Source: CAD feature listing. Evaluate the final solid. Frame: model axes, mm. Face numbers are marked on the shaded views. A direction names the side the tool comes from. Round coordinates to 2 decimals unless told otherwise and drop trailing zeros. Order: outer loops, then holes, each group sorted by start corner. A loop starts at its lowest first (then second) coordinate and runs counter-clockwise, first axis right, second up. Notation, with made-up numbers: (54, 23) - (113, 23) arc R13 ccw to (113, 37) - close; hole circle Ø5 at (74.5, 73.25). An arc over 180 degrees is marked (long way). Return JSON: item names as keys, results as strings. Group by question number.
1) Ray query, line 1 (X direction, y = 12, z = -7); line 2 (X direction, y = 3, z = 60). Return the intervals inside material, ascending. Write a range as from..to.
2) Mould query, pull axis Z, two halves, no side actions, for the marked faces 1, 2 and 3. Classes: pulls with the +Z half, pulls with the -Z half, needs draft (parallel to the pull), parting line crosses it, or undercut.
3) Section C-C, the plane y = 27.5. Return loops of the section in (x, z), plus the area to 3 significant figures.
4) Section B-B, the plane x = 40. Return loops of the section in (y, z).
5) Contact query for flat-ended pins moving along their axis: P1, Ø12, axis at x = -40, z = -59, coming from the +Y side; P2, Ø1, axis at x = 7, z = -39, coming from the -Y side; P3, Ø2, axis at x = -4.5, y = 23, coming from the -Z side. Output: stop coordinate, or through.
6) Section A-A, the plane z = 60. Return loops of the section in (x, y), plus the area to 3 significant figures.
7) Section D-D, the plane z = -18. Return loops of the section in (x, y).
8) Access query for the marked faces 4 and 5. Directions: +Z, -Z, +X, -X, +Y, -Y. A direction counts if a zero-diameter tool reaches every point of the face in a straight line with its end or side. Return the directions, or none.
```python
from build123d import *

# Parameters (mm, degrees)
SKETCH1_W               = 100
SKETCH1_H               = 100
BOSS_EXTRUDE1_DEPTH     = 50
SKETCH2_W               = 92
SKETCH2_H               = 92
CUT_EXTRUDE1_DEPTH      = 48
CUT_EXTRUDE2_DEPTH      = 123.474487139
CUT_EXTRUDE2_DEPTH_BACK = 123.474487139
SKETCH6_W               = 10
SKETCH6_H               = 5
SKETCH3_W               = 20
SKETCH3_H               = 40
BOSS_EXTRUDE2_DEPTH     = 15
BOSS_EXTRUDE3_START     = -43
SKETCH5_R               = 1.5
BOSS_EXTRUDE3_DEPTH     = 48
MIRROR2_COPY_1_SKETCH_W = 20
MIRROR2_COPY_1_SKETCH_H = 40
MIRROR2_COPY_1_DEPTH    = 15
MIRROR2_START           = -43
MIRROR2_COPY_2_SKETCH_R = 1.5
MIRROR2_COPY_2_DEPTH    = 48


with BuildPart() as part:
    # Sketch1 → Boss-Extrude1 (new body)
    with BuildSketch(Plane(origin=(0, 0, 0), x_dir=(1, 0, 0), z_dir=(0, 1, 0))):
        Rectangle(SKETCH1_W, SKETCH1_H)
    extrude(amount=BOSS_EXTRUDE1_DEPTH)

    # Sketch2 → Cut-Extrude1 (cut)
    with BuildSketch(Plane(origin=(0, 50, 0), x_dir=(1, 0, 0), z_dir=(0, 1, 0))):
        Rectangle(SKETCH2_W, SKETCH2_H)
    extrude(amount=-CUT_EXTRUDE1_DEPTH, mode=Mode.SUBTRACT)

    # Sketch6 → Cut-Extrude2 (cut, two sides: drawn at the far end of the back side and taken through both)
    with BuildSketch(Plane.XY.offset(50).offset(-CUT_EXTRUDE2_DEPTH_BACK)):
        with Locations((-25, 6.5)):
            Rectangle(SKETCH6_W, SKETCH6_H)
        with Locations((25, 6.5)):
            Rectangle(SKETCH6_W, SKETCH6_H)
    extrude(amount=CUT_EXTRUDE2_DEPTH + CUT_EXTRUDE2_DEPTH_BACK, mode=Mode.SUBTRACT)

    # Sketch3 → Boss-Extrude2 (add)
    with BuildSketch(Plane.XY.offset(50)):
        with Locations((-40, 20)):
            Rectangle(SKETCH3_W, SKETCH3_H)
    boss_extrude2 = extrude(amount=BOSS_EXTRUDE2_DEPTH)

    # Sketch5 → Boss-Extrude3 (add)
    with BuildSketch(Plane(origin=(0, 40, 0), x_dir=(1, 0, 0), z_dir=(0, 1, 0)).offset(BOSS_EXTRUDE3_START)):
        with Locations(Location((-40, -60, 0), (0, 0, 270))):
            Circle(SKETCH5_R)
    boss_extrude3 = extrude(amount=BOSS_EXTRUDE3_DEPTH)

    # Mirror1: Boss-Extrude2, Boss-Extrude3 across plane
    add(boss_extrude2.mirror(Plane.ZY))
    add(boss_extrude3.mirror(Plane.ZY))

    # Mirror2: Boss-Extrude2, Boss-Extrude3 across plane
    add(boss_extrude2.mirror(Plane(origin=(0, 0, 0), x_dir=(1, 0, 0), z_dir=(0, 0, -1))))
    add(boss_extrude3.mirror(Plane(origin=(0, 0, 0), x_dir=(1, 0, 0), z_dir=(0, 0, -1))))

    # Mirror2 copy 1 sketch → Mirror2 copy 1 (add)
    with BuildSketch(Plane(origin=(0, 0, -50), x_dir=(-1, 0, 0), z_dir=(0, 0, -1))):
        with Locations((-40, 20)):
            Rectangle(MIRROR2_COPY_1_SKETCH_W, MIRROR2_COPY_1_SKETCH_H)
    extrude(amount=MIRROR2_COPY_1_DEPTH)

    # Mirror2 copy 2 sketch → Mirror2 copy 2 (add)
    with BuildSketch(Plane(origin=(0, 40, 0), x_dir=(-1, 0, 0), z_dir=(0, 1, 0)).offset(MIRROR2_START)):
        with Locations(Location((-40, -60, 0), (0, 0, 270))):
            Circle(MIRROR2_COPY_2_SKETCH_R)
    extrude(amount=MIRROR2_COPY_2_DEPTH)


solid = part.part
```
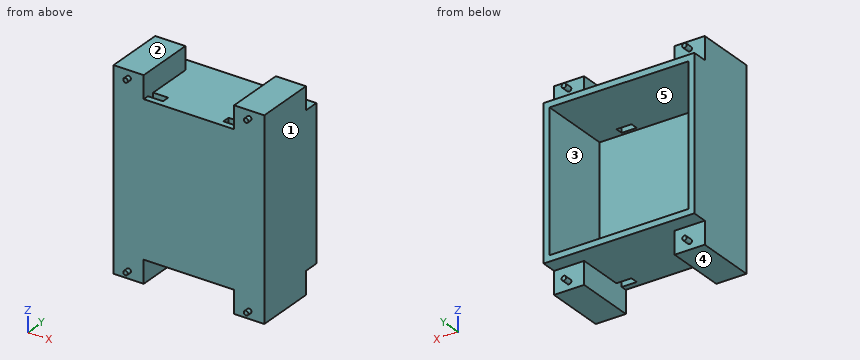
Geometry check:
{
 "1": {"line 1": "-50..-46, 46..50", "line 2": "-50..-30, 30..50"},
 "2": {"face 1": "needs draft", "face 2": "pulls with the +Z half", "face 3": "undercut"},
 "3": {"outline": "(-50, -65) - (-30, -65) - (-30, -50) - (30, -50) - (30, -65) - (50, -65) - (50, 65) - (30, 65) - (30, 50) - (-30, 50) - (-30, 65) - (-50, 65) - close; hole (-46, -46) - (46, -46) - (46, 46) - (-46, 46) - close", "area": "2,740 mm2"},
 "4": {"outline": "(-3, -61.5) - (0, -61.5) - (0, -65) - (40, -65) - (40, -61.5) - (45, -61.5) - (45, -58.5) - (40, -58.5) - (40, -50) - (50, -50) - (50, -46) - (2, -46) - (2, 46) - (50, 46) - (50, 50) - (40, 50) - (40, 58.5) - (45, 58.5) - (45, 61.5) - (40, 61.5) - (40, 65) - (0, 65) - (0, 61.5) - (-3, 61.5) - (-3, 58.5) - (0, 58.5) - (0, -58.5) - (-3, -58.5) - close"},
 "5": {"P1": "y = 45", "P2": "y = 0", "P3": "z = -50"},
 "6": {"outline": "(-50, 0) - (-41.5, 0) - (-41.5, -3) - (-38.5, -3) - (-38.5, 0) - (-30, 0) - (-30, 40) - (-38.5, 40) - (-38.5, 45) - (-41.5, 45) - (-41.5, 40) - (-50, 40) - close; (30, 0) - (38.5, 0) - (38.5, -3) - (41.5, -3) - (41.5, 0) - (50, 0) - (50, 40) - (41.5, 40) - (41.5, 45) - (38.5, 45) - (38.5, 40) - (30, 40) - close", "area": "1,650 mm2"},
 "7": {"outline": "(-50, 0) - (50, 0) - (50, 50) - (46, 50) - (46, 2) - (-46, 2) - (-46, 50) - (-50, 50) - close"},
 "8": {"face 4": "-Z, +X, -X, +Y, -Y", "face 5": "+Y"}
}
